The listing builds one solid part. Answer for the finished solid, in the listing's coordinates (mm). Face numbers are marked on the shaded views. A direction names the side the tool comes from. Round coordinates to 2 decimals unless told otherwise and drop trailing zeros. Write each loop counter-clockwise with the first axis right and the second up, starting at its lowest first coordinate (ties: lowest second). Pieces come first, ordered by that corner, then holes. Notation, with made-up numbers: M -0.75,-17 L 6.25,-17 A21 cw 6.25,21 Z; hole C 35,-12.75 d3. An arc over 180 degrees is marked long. Write each question's results on one line, items separated by ' | '.
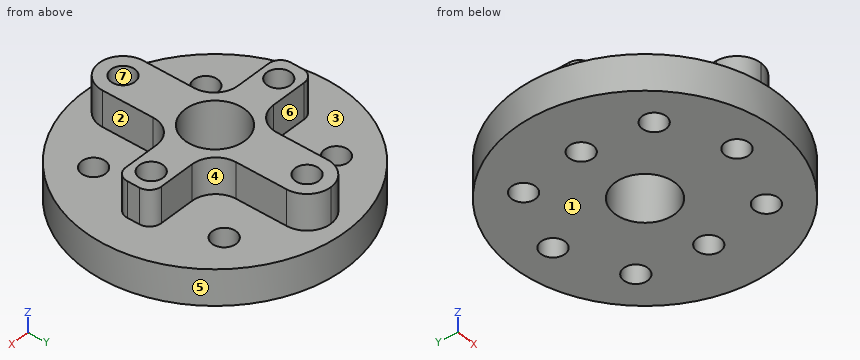
from build123d import *

# Parameters (mm, degrees)
F0_R     = 1
F0_R_2   = 2.5
F1_DEPTH = 3
F2_R     = 11
F2_R_2   = 1
F2_R_3   = 2.5
F3_DEPTH = 3


with BuildPart() as f1:
    # F0 (on Top) → F1 (new body)
    with BuildSketch(Plane.XY):
        with BuildLine():
            ThreePointArc((4, 1.5), (2.5857864376, 2.0857864376), (2, 3.5))
            Line((2, 3.5), (2, 7.75))
            ThreePointArc((2, 7.75), (1.4142135624, 9.1642135624), (0, 9.75))
            ThreePointArc((0, 9.75), (-1.4142135624, 9.1642135624), (-2, 7.75))
            Line((-2, 7.75), (-2, 3.5))
            ThreePointArc((-2, 3.5), (-2.5857864376, 2.0857864376), (-4, 1.5))
            Line((-4, 1.5), (-7, 1.5))
            ThreePointArc((-7, 1.5), (-7.7071067812, 1.2071067812), (-8, 0.5))
            Line((-8, 0.5), (-8, -0.5))
            ThreePointArc((-8, -0.5), (-7.7071067812, -1.2071067812), (-7, -1.5))
            Line((-7, -1.5), (-4, -1.5))
            ThreePointArc((-4, -1.5), (-2.5857864376, -2.0857864376), (-2, -3.5))
            Line((-2, -3.5), (-2, -7.75))
            ThreePointArc((-2, -7.75), (-1.4142135624, -9.1642135624), (0, -9.75))
            ThreePointArc((0, -9.75), (1.4142135624, -9.1642135624), (2, -7.75))
            Line((2, -7.75), (2, -3.5))
            ThreePointArc((2, -3.5), (2.5857864376, -2.0857864376), (4, -1.5))
            Line((4, -1.5), (7, -1.5))
            ThreePointArc((7, -1.5), (7.7071067812, -1.2071067812), (8, -0.5))
            Line((8, -0.5), (8, 0.5))
            ThreePointArc((8, 0.5), (7.7071067812, 1.2071067812), (7, 1.5))
            Line((7, 1.5), (4, 1.5))
        make_face()
        with Locations((0, -7.75)):
            Circle(F0_R, mode=Mode.SUBTRACT)
        with Locations((-6.25, 0)):
            Circle(F0_R, mode=Mode.SUBTRACT)
        Circle(F0_R_2, mode=Mode.SUBTRACT)
        with Locations((6.25, 0)):
            Circle(F0_R, mode=Mode.SUBTRACT)
        with Locations((0, 7.75)):
            Circle(F0_R, mode=Mode.SUBTRACT)
    extrude(amount=F1_DEPTH)

    # F2 (on face) → F3 (join)
    with BuildSketch(Plane(origin=(0, 0, 0), x_dir=(1, 0, 0), z_dir=(0, 0, -1))):
        Circle(F2_R)
        with Locations((-5.5, -5.5)):
            Circle(F2_R_2, mode=Mode.SUBTRACT)
        with Locations((5.5, -5.5)):
            Circle(F2_R_2, mode=Mode.SUBTRACT)
        with Locations((-5.5, 5.5)):
            Circle(F2_R_2, mode=Mode.SUBTRACT)
        with BuildLine():
            ThreePointArc((-2, 7.75), (0, 9.75), (2, 7.75))
            Line((2, 7.75), (2, 3.5))
            ThreePointArc((2, 3.5), (2.5857864376, 2.0857864376), (4, 1.5))
            Line((4, 1.5), (7, 1.5))
            ThreePointArc((7, 1.5), (7.7071067812, 1.2071067812), (8, 0.5))
            Line((8, 0.5), (8, -0.5))
            ThreePointArc((8, -0.5), (7.7071067812, -1.2071067812), (7, -1.5))
            Line((7, -1.5), (4, -1.5))
            ThreePointArc((4, -1.5), (2.5857864376, -2.0857864376), (2, -3.5))
            Line((2, -3.5), (2, -7.75))
            ThreePointArc((2, -7.75), (0, -9.75), (-2, -7.75))
            Line((-2, -7.75), (-2, -3.5))
            ThreePointArc((-2, -3.5), (-2.5857864376, -2.0857864376), (-4, -1.5))
            Line((-4, -1.5), (-7, -1.5))
            ThreePointArc((-7, -1.5), (-7.7071067812, -1.2071067812), (-8, -0.5))
            Line((-8, -0.5), (-8, 0.5))
            ThreePointArc((-8, 0.5), (-7.7071067812, 1.2071067812), (-7, 1.5))
            Line((-7, 1.5), (-4, 1.5))
            ThreePointArc((-4, 1.5), (-2.5857864376, 2.0857864376), (-2, 3.5))
            Line((-2, 3.5), (-2, 7.75))
        make_face(mode=Mode.SUBTRACT)
        with Locations((5.5, 5.5)):
            Circle(F2_R_2, mode=Mode.SUBTRACT)
        with BuildLine():
            Line((2, 3.5), (2, 7.75))
            ThreePointArc((2, 7.75), (0, 9.75), (-2, 7.75))
            Line((-2, 7.75), (-2, 3.5))
            ThreePointArc((-2, 3.5), (-2.5857864376, 2.0857864376), (-4, 1.5))
            Line((-4, 1.5), (-7, 1.5))
            ThreePointArc((-7, 1.5), (-7.7071067812, 1.2071067812), (-8, 0.5))
            Line((-8, 0.5), (-8, -0.5))
            ThreePointArc((-8, -0.5), (-7.7071067812, -1.2071067812), (-7, -1.5))
            Line((-7, -1.5), (-4, -1.5))
            ThreePointArc((-4, -1.5), (-2.5857864376, -2.0857864376), (-2, -3.5))
            Line((-2, -3.5), (-2, -7.75))
            ThreePointArc((-2, -7.75), (0, -9.75), (2, -7.75))
            Line((2, -7.75), (2, -3.5))
            ThreePointArc((2, -3.5), (2.5857864376, -2.0857864376), (4, -1.5))
            Line((4, -1.5), (7, -1.5))
            ThreePointArc((7, -1.5), (7.7071067812, -1.2071067812), (8, -0.5))
            Line((8, -0.5), (8, 0.5))
            ThreePointArc((8, 0.5), (7.7071067812, 1.2071067812), (7, 1.5))
            Line((7, 1.5), (4, 1.5))
            ThreePointArc((4, 1.5), (2.5857864376, 2.0857864376), (2, 3.5))
        make_face()
        with Locations((0, -7.75)):
            Circle(F2_R_2, mode=Mode.SUBTRACT)
        with Locations((-6.25, 0)):
            Circle(F2_R_2, mode=Mode.SUBTRACT)
        Circle(F2_R_3, mode=Mode.SUBTRACT)
        with Locations((6.25, 0)):
            Circle(F2_R_2, mode=Mode.SUBTRACT)
        with Locations((0, 7.75)):
            Circle(F2_R_2, mode=Mode.SUBTRACT)
    extrude(amount=F3_DEPTH)


solid = f1.part
1) Section A-A (y = 0) is taken. Determine the outline of the cut face in (x, z).
Return value:
outline: M -11,-3 L -7.25,-3 L -7.25,3 L -8,3 L -8,0 L -11,0 Z; M -5.25,-3 L -2.5,-3 L -2.5,3 L -5.25,3 Z; M 2.5,-3 L 5.25,-3 L 5.25,3 L 2.5,3 Z; M 7.25,-3 L 11,-3 L 11,0 L 8,0 L 8,3 L 7.25,3 Z
2) A tool of negligible diameter and unlimited length cuts with its end or side. For the marked faces 1, 2, 3 and 4, from which of +Z, -Z, +X, -X, +Y, -Y can it reach the whole face along a straight path? Write none if from no direction.
Return value:
face 1: -Z, +X, -X, +Y, -Y | face 2: +Z, +X, -Y | face 3: +Z | face 4: +Z, +X, +Y
3) Section B-B (z = 0.7) is taken. Determine the outline of the cut face in (x, y), then the cut area to 3 significant figures.
Return value:
outline: M -8,-0.5 A1 ccw -7,-1.5 L -4,-1.5 A2 cw -2,-3.5 L -2,-7.75 A2 ccw 2,-7.75 L 2,-3.5 A2 cw 4,-1.5 L 7,-1.5 A1 ccw 8,-0.5 L 8,0.5 A1 ccw 7,1.5 L 4,1.5 A2 cw 2,3.5 L 2,7.75 A2 ccw -2,7.75 L -2,3.5 A2 cw -4,1.5 L -7,1.5 A1 ccw -8,0.5 Z; hole C -6.25,0 d2; hole C 0,0 d5; hole C 0,-7.75 d2; hole C 0,7.75 d2; hole C 6.25,0 d2 | area: 80.9 mm²
4) Find the intervals of material crossed by line 1 (X direction, y = 0, z = 0.75); line 2 (Y direction, x = 0, z = -1.6); line 3 (X direction, y = 0, z = -0.5), in increasing order.
Return value:
line 1: -8 to -7.25, -5.25 to -2.5, 2.5 to 5.25, 7.25 to 8 | line 2: -11 to -8.75, -6.75 to -2.5, 2.5 to 6.75, 8.75 to 11 | line 3: -11 to -7.25, -5.25 to -2.5, 2.5 to 5.25, 7.25 to 11
5) Section C-C (x = -5.75) is taken. Determine the outline of the cut face in (y, z), then the cut area to 3 significant figures.
Return value:
outline: M -9.38,-3 L -6.47,-3 L -6.47,0 L -9.38,0 Z; M -4.53,-3 L -0.87,-3 L -0.87,3 L -1.5,3 L -1.5,0 L -4.53,0 Z; M 0.87,-3 L 4.53,-3 L 4.53,0 L 1.5,0 L 1.5,3 L 0.87,3 Z; M 6.47,-3 L 9.38,-3 L 9.38,0 L 6.47,0 Z | area: 43.3 mm²
6) Each of these flat-tipped pins is pushed along its axis until it touches: pin 1 (0.5 mm diameter, centred on y = 0, z = 1, fed in from -X); pin 2 (2.5 mm diameter, centred on x = 5, z = 2, fed in from +Y); pin 3 (1.8 mm diameter, centred on x = -6.25, y = 0, fed in from -Z); pin 4 (0.5 mm diameter, centred on y = 0, z = 1.5, fed in from +X). Where does it stop, or does it pass through?
Return value:
pin 1: x = -8 | pin 2: y = 1.52 | pin 3: through | pin 4: x = 8
7) The mould has two halves that part along X. Classify the marked faces 5, 6 and 7: +X half, -X half, draft (parallel to the pull), parting line (faces both ways), or undercut.
Return value:
face 5: parting line | face 6: draft | face 7: undercut
8) Section D-D (z = -2.45) is taken. State how many separate pieces and enclosed holes the cut face has, then the cut area to 3 significant figures.
Return value:
separate pieces: 1 | enclosed holes: 9 | area: 335 mm²
